For this review, take the finished solid that the model builds, in its own axes (mm). A direction names the side the tool comes from. Give positions to 0.01 mm unless a question says otherwise; leave off trailing zeros. Loops run counter-clockwise (first coordinate to the right, second up) from the corner with the lowest first, then second, coordinate; pieces in that order, holes last.
```python
from build123d import *

# Parameters (mm, degrees)
CHAMFER_SIZE = 0.25


with BuildPart() as part:
    # Sketch → Revolution (revolve)
    with BuildSketch(Plane.XZ):
        Polygon((4, -3.5), (6.5, -3.5), (6.75, -3.25), (9, -3.25), (9.25, -3.5), (11, -3.5), (11, 3.5), (9.25, 3.5), (9, 3.25), (6.75, 3.25), (6.5, 3.5), (4, 3.5), align=None)
    revolve(axis=Axis((0, 0, 0), (0, 0, 1)))

    # Chamfer
    chamfer_edges = [part.edges().sort_by_distance(p)[0] for p in [
        (-11, 0, -3.5),
        (-4, 0, -3.5),
        (-11, 0, 3.5),
        (-4, 0, 3.5),
    ]]
    chamfer(chamfer_edges, length=CHAMFER_SIZE)


solid = part.part
```
Q1. Machinability: for faces 4 (the cylindrical face through (-0.867, -3.905, -0.046)), 5 (the flat face through (1, 7, 3.25)), which of the approach directions +Z, -Z, +X, -X, +Y, -Y give a long, thin tool a straight path to every point of the face, cutting with its end or side? Answer none if there is none.
Answers:
face 4: +Z, -Z
face 5: +Z
Q2. For pin 1 Ø1.5 at (x, y) = (3.5, 6.5) entering from -Z; pin 2 Ø4 at (y, z) = (-8, -0.5) entering from -X; pin 3 Ø3 at (y, z) = (-3, 2) entering from -X, all flat-tipped, find the tip position at first contact; note any pin that passes through.
Answers:
pin 1: stops at z = -3.37
pin 2: stops at x = -9.22
pin 3: stops at x = -10.9
Q3. For probe 1 along Y at (x, z) = (0, 0); probe 2 along Z at (x, y) = (-1.25, -8); probe 3 along X at (y, z) = (0.75, -2.5), list the stretches that pass through material, from the lowest coordinate up.
Answers:
probe 1: y = -11 to -4, 4 to 11
probe 2: z = -3.25 to 3.25
probe 3: x = -10.97 to -3.93, 3.93 to 10.97
Q4. Mouldability with a two-part tool opening along X and no side actions: class faces 1 (the flat face through (-1, 7, -3.25)), 2 (the cylindrical face through (-2.38, -10.74, 0.05)), 3 (the flat face through (-5, 8, -3.5)) as +X half, -X half, draft (parallel to the pull), parting line (faces both ways), or undercut.
Answers:
face 1: undercut
face 2: parting line
face 3: draft
Q5. Consider section C-C on z = -1.75. Give the boundary of the cut face in (x, y).
Answers:
outline: circle Ø22 at (0, 0); hole circle Ø8 at (0, 0)
